Geometry: final body of the model. Coordinates: model frame, mm. A direction names the side the tool comes from. Give positions to 0.01 mm unless a question says otherwise; leave off trailing zeros. Order: outer loops, then holes, each group sorted by start corner. A loop starts at its lowest first (then second) coordinate and runs counter-clockwise, first axis right, second up. Notation, with made-up numbers: (28.5, -14) - (49.5, -14) arc R27 ccw to (49.5, 17) - close; hole circle Ø4 at (-22, 59.25). An arc over 180 degrees is marked (long way). Write item = value, one per line. Start each with the question number.
from build123d import *

# Parameters (mm, degrees)
F0_W     = 1200
F0_H     = 18
F1_DEPTH = 600
F2_W     = 18
F2_H     = 1097
F3_DEPTH = 500
F4_W     = 964
F4_H     = 18
F5_DEPTH = 500
F6_W     = 964
F6_H     = 300
F7_DEPTH = 18


with BuildPart() as f1:
    # F0 (on Front) → F1 (new body)
    with BuildSketch(Plane.XZ):
        with Locations((0, 1106)):
            Rectangle(F0_W, F0_H)
    extrude(amount=F1_DEPTH)

    # F2 (on Front) → F3 (join)
    with BuildSketch(Plane.XZ):
        with Locations((-491, 548.5)):
            Rectangle(F2_W, F2_H)
        with Locations((491, 548.5)):
            Rectangle(F2_W, F2_H)
    extrude(amount=F3_DEPTH)

    # F4 (on Front) → F5 (join)
    with BuildSketch(Plane.XZ):
        with Locations((0, 191)):
            Rectangle(F4_W, F4_H)
        with Locations((0, 584)):
            Rectangle(F4_W, F4_H)
        with Locations((0, 902)):
            Rectangle(F4_W, F4_H)
    extrude(amount=F5_DEPTH)

    # F6 (on Front) → F7 (join)
    with BuildSketch(Plane.XZ):
        with Locations((0, 743)):
            Rectangle(F6_W, F6_H)
    extrude(amount=F7_DEPTH)


solid = f1.part
Q1. Section B-B, the plane y = -65. Return the cut outline in (x, z).
Q2. Section A-A, the plane z = 485. Return the cut outline in (x, y).
Q3. Material intervals for line 1 along Z through (x, y) = (-332, -471.5); line 2 along X through (y, z) = (-160, 821.5); line 3 along Y through (x, z) = (430.5, 832.5), sorted ascending. Write a range as from..to.
Q4. Contact query for flat-ended pins moving along their axis: pin 1 (1 mm diameter, centred on x = 439, z = 772, fed in from -Y); pin 2 (8 mm diameter, centred on y = -226, z = 161, fed in from -X); pin 3 (12 mm diameter, centred on y = -134, z = 143.5, fed in from +X). Output: stop coordinate, or through.
Q5. Section D-D, the plane y = -541.5. Return the cut outline in (x, z), then the cut area to 3 significant figures.
Q6. Set-up query: faces 5 (the flat face through (-7, -246, 200)), 6 (the flat face through (-7, -256, 893)), 7 (the flat face through (482, -246, 90)). Return all of +Z, -Z, +X, -X, +Y, -Y with unobstructed straight access to the full face (end or side cutting, diameter ignored); none if empty.
Q7. Pull-direction query (X, two-part tool) for faces 1 (the flat face through (-482, -246, 90)), 2 (the flat face through (-500, -246, 541)), 3 (the flat face through (-150, -500, 592)), 4 (the flat face through (500, -246, 541)); classes: +X half, -X half, draft (parallel to the pull), parting line (faces both ways), or undercut.
Q8. Section C-C, the plane x = -334. Return the cut outline in (y, z).
The answers:
q1.outline = (-600, 1097) - (-500, 1097) - (-500, 0) - (-482, 0) - (-482, 182) - (482, 182) - (482, 0) - (500, 0) - (500, 1097) - (600, 1097) - (600, 1115) - (-600, 1115) - close; hole (-482, 200) - (482, 200) - (482, 575) - (-482, 575) - close; hole (-482, 593) - (482, 593) - (482, 893) - (-482, 893) - close; hole (-482, 911) - (482, 911) - (482, 1097) - (-482, 1097) - close
q2.outline = (-500, -500) - (-482, -500) - (-482, 0) - (-500, 0) - close; (482, -500) - (500, -500) - (500, 0) - (482, 0) - close
q3.line_1 = 182..200, 575..593, 893..911, 1097..1115
q3.line_2 = -500..-482, 482..500
q3.line_3 = -18..0
q4.pin_1 = -18
q4.pin_2 = -500
q4.pin_3 = 500
q5.outline = (-600, 1097) - (600, 1097) - (600, 1115) - (-600, 1115) - close
q5.area = 21,600 mm²
q6.face_5 = +Y, -Y
q6.face_6 = -Y
q6.face_7 = -Z, +Y, -Y
q7.face_1 = undercut
q7.face_2 = -X half
q7.face_3 = draft
q7.face_4 = +X half
q8.outline = (-600, 1097) - (0, 1097) - (0, 1115) - (-600, 1115) - close; (-500, 182) - (0, 182) - (0, 200) - (-500, 200) - close; (-500, 575) - (0, 575) - (0, 911) - (-500, 911) - (-500, 893) - (-18, 893) - (-18, 593) - (-500, 593) - close
